Input: part model. Units: mm. Frame: model coordinates. A direction names the side the tool comes from. Round coordinates to 2 decimals unless told otherwise and drop trailing zeros. Order: outer loops, then holes, each group sorted by start corner. A loop starts at its lowest first (then second) coordinate and runs counter-clockwise, first axis right, second up. Notation, with made-up numbers: (28.5, 13.5) -> (34.5, 13.5) arc R5 ccw to (34.5, 18.5) -> close; hole circle Ø6 at (38, 76.5). An arc over 180 degrees is marked (long way). Use a Markdown table: item, result.
from build123d import *

# Parameters (mm, degrees)
SKETCH1_R           = 4.25
BOSS_EXTRUDE1_DEPTH = 71.68750559
CUT_EXTRUDE1_DEPTH  = 6.6
CHAMFER1_SIZE       = 0.5
CUT_EXTRUDE2_DEPTH  = 6.6
CHAMFER2_SIZE       = 0.5


with BuildPart() as part:
    # Sketch1 → Boss-Extrude1 (new body)
    with BuildSketch(Plane(origin=(0, 0, 0), x_dir=(1, 0, 0), z_dir=(0, 1, 0))):
        Circle(SKETCH1_R)
    extrude(amount=BOSS_EXTRUDE1_DEPTH)

    # Sketch2 → Cut-Extrude1 (cut)
    with BuildSketch(Plane(origin=(0, 71.68750559, 0), x_dir=(1, 0, 0), z_dir=(0, 1, 0))):
        Polygon((1.616580754, 2.8), (-1.616580754, 2.8), (-3.233161507, 0), (-1.616580754, -2.8), (1.616580754, -2.8), (3.233161507, 0), align=None)
    extrude(amount=-CUT_EXTRUDE1_DEPTH, mode=Mode.SUBTRACT)

    # Chamfer1
    chamfer1_edges = [part.edges().sort_by_distance(p)[0] for p in [
        (2.424871131, 71.68750559, -1.4),
        (0, 71.68750559, -2.8),
        (-2.424871131, 71.68750559, -1.4),
        (-2.424871131, 71.68750559, 1.4),
        (0, 71.68750559, 2.8),
        (2.424871131, 71.68750559, 1.4),
    ]]
    chamfer(chamfer1_edges, length=CHAMFER1_SIZE)

    # Sketch3 → Cut-Extrude2 (cut)
    with BuildSketch(Plane.XZ):
        Polygon((0, 3.233161507), (-2.8, 1.616580754), (-2.8, -1.616580754), (0, -3.233161507), (2.8, -1.616580754), (2.8, 1.616580754), align=None)
    extrude(amount=-CUT_EXTRUDE2_DEPTH, mode=Mode.SUBTRACT)

    # Chamfer2
    chamfer2_edges = [part.edges().sort_by_distance(p)[0] for p in [
        (1.4, 0, 2.424871131),
        (-1.4, 0, 2.424871131),
        (-2.8, 0, 0),
        (-1.4, 0, -2.424871131),
        (1.4, 0, -2.424871131),
        (2.8, 0, 0),
    ]]
    chamfer(chamfer2_edges, length=CHAMFER2_SIZE)


solid = part.part
1) Contact query for a flat-ended pin moving along its axis: P1, Ø1.7, axis at x = -1, z = 1.5, coming from the -Y side. Output: stop coordinate, or through.
Answer key:
| item | result |
|---|---|
| P1 | stops at y = 6.6 |
2) Draft query along X for faces 1 (the face through (2.436, 68.18, -1.38)), 2 (the face through (-3, 71.688, -2)), 3 (the face through (2.285, 35.342, -3.584)), 4 (the face through (-1.42, 3.507, -2.414)). Return one class per face: released by +X, released by -X, zero draft, split by the parting line, or undercut.
Answer key:
| item | result |
|---|---|
| face 1 | undercut |
| face 2 | zero draft |
| face 3 | split by the parting line |
| face 4 | undercut |
3) Cut plane C-C on z = -1. Return loops of the section in (x, y).
Answer key:
| item | result |
|---|---|
| outline | (-4.13, 0) -> (-3.3, 0) -> (-2.8, 0.5) -> (-2.8, 6.6) -> (2.8, 6.6) -> (2.8, 0.5) -> (3.3, 0) -> (4.13, 0) -> (4.13, 71.69) -> (3.23, 71.69) -> (2.66, 71.19) -> (2.66, 65.09) -> (-2.66, 65.09) -> (-2.66, 71.19) -> (-3.23, 71.69) -> (-4.13, 71.69) -> close |
4) Cut plane B-B on y = 45. Return loops of the section in (x, z).
Answer key:
| item | result |
|---|---|
| outline | circle Ø8.5 at (0, 0) |
5) Ray query, probe 1 along Y at (x, z) = (-1.5, 0); probe 2 along X at (y, z) = (43, 0.25); probe 3 along Z at (x, y) = (-2.75, 32.5). Return the intervals inside material, ascending.
Answer key:
| item | result |
|---|---|
| probe 1 | y = 6.6 to 65.09 |
| probe 2 | x = -4.24 to 4.24 |
| probe 3 | z = -3.24 to 3.24 |
6) Set-up query: faces 5 (the face through (2.65, 71.43, -1.5)), 6 (the face through (-2.8, 4, 0)). Return all of +Z, -Z, +X, -X, +Y, -Y with unobstructed straight access to the full face (end or side cutting, diameter ignored); none if empty.
Answer key:
| item | result |
|---|---|
| face 5 | +Y |
| face 6 | -Y |
7) Cut plane A-A on x = -1. Return loops of the section in (y, z), and give its area (3 significant figures).
Answer key:
| item | result |
|---|---|
| outline | (0, -4.13) -> (71.69, -4.13) -> (71.69, -3.3) -> (71.19, -2.8) -> (65.09, -2.8) -> (65.09, 2.8) -> (71.19, 2.8) -> (71.69, 3.3) -> (71.69, 4.13) -> (0, 4.13) -> (0, 3.23) -> (0.5, 2.66) -> (6.6, 2.66) -> (6.6, -2.66) -> (0.5, -2.66) -> (0, -3.23) -> close |
| area | 520 mm^2 |
